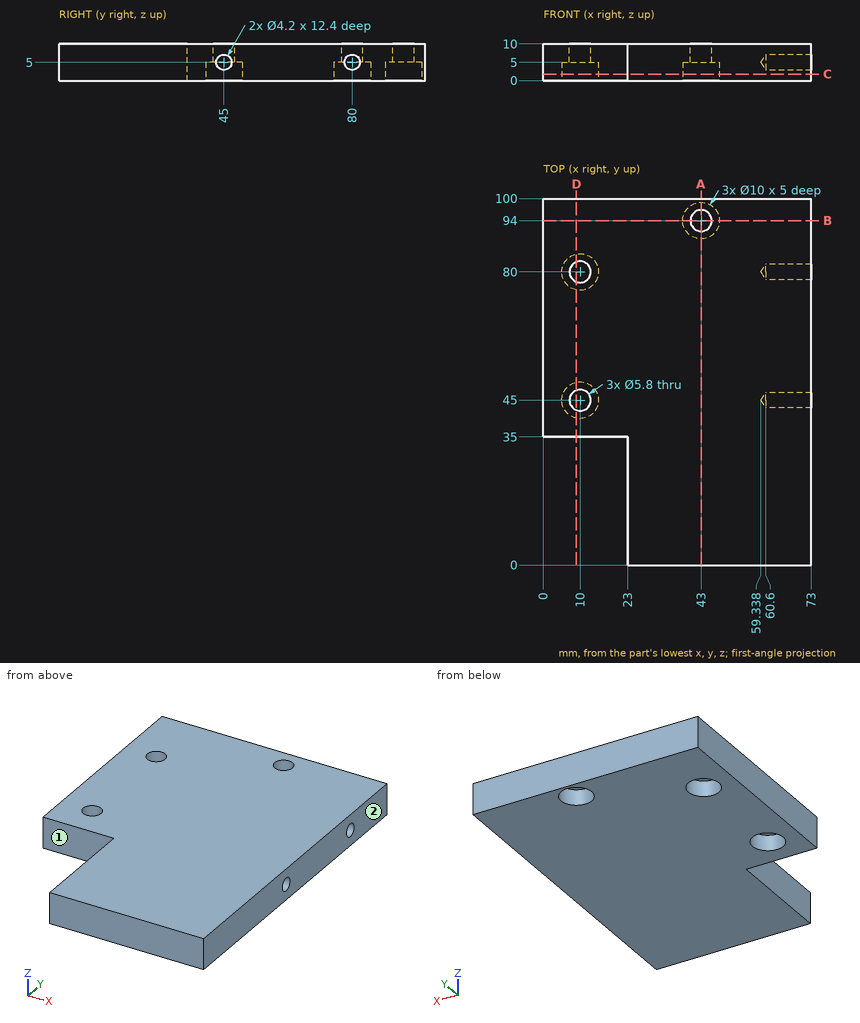
Geometry: see drawing. Coordinates: mm, zero at the bounding-box minimum. A direction names the side the tool comes from. Give positions to 0.01 mm unless a question says otherwise; leave off trailing zeros. Loops run counter-clockwise (first coordinate to the right, second up) from the corner with the lowest first, then second, coordinate; pieces in that order, holes last. Notation, with made-up numbers: M -6,-36.5 L 13,-36.5 A12 cw 13,-23.5 Z; hole C -11.5,82.25 d9. An arc over 180 degrees is marked long. Use one line per item in the form item = value.
1. Section query B-B, the plane y = 94. Return the cut outline in (x, z).
Numbers:
outline = M 0,0 L 38,0 L 38,5 L 40.1,5 L 40.1,10 L 0,10 Z; M 45.9,5 L 48,5 L 48,0 L 73,0 L 73,10 L 45.9,10 Z
2. Section query C-C, the plane z = 1.75. Return the cut outline in (x, y), and give its area (3 significant figures).
Numbers:
outline = M 0,35 L 23,35 L 23,0 L 73,0 L 73,100 L 0,100 Z; hole C 10,45 d10; hole C 10,80 d10; hole C 43,94 d10
area = 6,260 mm²
3. Section query A-A, the plane x = 43. Return the cut outline in (y, z).
Numbers:
outline = M 0,0 L 89,0 L 89,5 L 91.1,5 L 91.1,10 L 0,10 Z; M 96.9,5 L 99,5 L 99,0 L 100,0 L 100,10 L 96.9,10 Z
4. Reachability of the marked faces 1 and 2 from +Z, -Z, +X, -X, +Y, -Y: full face, straight path, thin tool, end or side. Return the list, or none.
Numbers:
face_1 = +Z, -Z, -X, -Y
face_2 = +Z, -Z, +X, +Y, -Y
5. Line query: L1, parallel to Y at x = 10, z = 2.3; L2, parallel to Y at x = 65, z = 5; L3, parallel to Z at x = 64.5, y = 45. Output: solid intervals per line, ascending.
Numbers:
L1 = 35 to 40, 50 to 75, 85 to 100
L2 = 0 to 42.9, 47.1 to 77.9, 82.1 to 100
L3 = 0 to 2.9, 7.1 to 10
6. Section query D-D, the plane x = 9. Return the cut outline in (y, z).
Numbers:
outline = M 35,0 L 40.1,0 L 40.1,5 L 42.28,5 L 42.28,10 L 35,10 Z; M 47.72,5 L 49.9,5 L 49.9,0 L 75.1,0 L 75.1,5 L 77.28,5 L 77.28,10 L 47.72,10 Z; M 82.72,5 L 84.9,5 L 84.9,0 L 100,0 L 100,10 L 82.72,10 Z
7. First-contact query: pin 1 (4 mm diameter, centred on y = 45, z = 5, fed in from +X); pin 2 (9 mm diameter, centred on x = 10, y = 80, fed in from -Z); pin 3 (5 mm diameter, centred on y = 13, z = 4, fed in from -X). Flat tips, straight axial feed; report the tip coordinate or a pass-through.
Numbers:
pin_1 = 60.54
pin_2 = 5
pin_3 = 23
